Input: part model. Units: mm. Frame: model coordinates. A direction names the side the tool comes from. Give positions to 0.01 mm unless a question says otherwise; leave off trailing zeros. Loops run counter-clockwise (first coordinate to the right, second up) from the corner with the lowest first, then second, coordinate; pieces in that order, holes last. Notation, with made-up numbers: M 43.5,79 L 51.5,79 A37 cw 51.5,117 Z; hole C 39,24.25 d10. An arc over 180 degrees is marked long. Answer as a JSON object with one key per item and string values. Group by question number.
1) Section query D-D on z = 15. Return loops of the section in (x, y), plus the area to 3 significant figures.
2) First-contact query: P1, Ø5.5, axis at y = 0, z = 0, coming from the -X side (3 decimals); P2, Ø3.5, axis at x = 2, y = 3.5, coming from the -Z side; P3, Ø3, axis at x = -1, z = -16.5, coming from the -Y side; P4, Ø3.5, axis at x = 0, z = 15, coming from the -Y side. Flat tips, straight axial feed; report the tip coordinate or a pass-through.
3) Section query C-C on x = 4.25. Return loops of the section in (y, z), plus the area to 3 significant figures.
4) Section query B-B on z = 0. Return loops of the section in (x, y).
5) Section query A-A on x = 0. Return loops of the section in (y, z).
6) Ray query, L1, parallel to Z at x = 0, y = 14.7; L2, parallel to Z at x = 3.5, y = 0; L3, parallel to X at y = 14.8, z = 15. Return the intervals inside material, ascending.
7) Draft query along X for faces 5 (the flat face through (6, 7, 0)), 6 (the flat face through (1, 16, -20)), 7 (the flat face through (0, 16, -17)). Return one class per face: +X half, -X half, draft (parallel to the pull), parting line (faces both ways), or undercut.
8) Access query for faces 1 (the flat face through (3, 14, 14)), 2 (the cylindrical face through (0.18, 5.9, -3.07)), 3 (the flat face through (0, 7, -10)), 4 (the flat face through (0, 16, 13)). Directions: +Z, -Z, +X, -X, +Y, -Y. A direction counts if a zero-diameter tool reaches every point of the face in a straight line with its end or side. Return the directions, or none.
Autodesk Inventor part; units mm, degrees
ref_plane "YZ Plane" through (0, 0, 0) normal (1, 0, 0) x (0, 1, 0)
ref_plane "XZ Plane" through (0, 0, 0) normal (0, 1, 0) x (-1, 0, 0)
ref_plane "XY Plane" through (0, 0, 0) normal (0, 0, 1) x (1, 0, 0)
sketch "Sketch1" plane through (0, 0, 0) normal (1, 0, 0) x (0, 1, 0)
  line L0 (0, 0) -> (14, 0) construction
  line L1 (0, -10) -> (14, -10)
  line L2 (14, 10) -> (0, 10)
  arc A0 (0, 10) -> (0, -10) centre (0, 0) ccw
  arc A1 (14, -10) -> (14, 10) centre (14, 0) ccw construction
  line L3 (14, 10) -> (14, -10)
  point P0 (7, 0)
  dimension "d2" = 20
  dimension "d1" = 14
extrude "Extrusion1" add sketch "Sketch1" along normal mid plane 10
sketch "Sketch2" plane through (-5, 14, 10) normal (0, 1, 0) x (1, 0, 0)
  line L0 (0, -10) -> (10, -10)
  line L1 (10, -10) -> (10, 30)
  line L2 (10, 30) -> (0, 30)
  line L3 (0, 30) -> (0, -10)
  line L4 (0, 0) -> (0, 20) construction
  line L5 (0, 20) -> (10, 20) construction
  line L6 (10, 20) -> (10, 0) construction
  line L7 (10, 0) -> (0, 0) construction
  line L8 (0, 0) -> (0, 20) construction
  line L9 (10, 20) -> (10, 0) construction
  line L10 (0, 10) -> (10, 10) construction
  point P0 (5, 10)
  dimension "d28" = 40
extrude "Extrusion2" add sketch "Sketch2" along normal blind 4
sketch "Sketch3" plane through (-5, 14, 10) normal (0, -1, 0) x (1, 0, 0)
  line L0 (10, -30) -> (0, -30)
  line L1 (0, -30) -> (0, -20)
  line L2 (0, -20) -> (0, 0)
  line L3 (0, 0) -> (0, 10)
  line L4 (0, 10) -> (10, 10)
  line L5 (10, 10) -> (10, 0)
  line L6 (10, 0) -> (10, -20)
  line L7 (10, -20) -> (10, -30)
  line L8 (10, -20) -> (0, -20)
  line L9 (0, 0) -> (10, 0)
  line L10 (0, 10) -> (10, 10)
  point P0 (5, -10)
  point P1 (5, 5)
  point P2 (5, -25)
  point P3 (5, 10)
  point P4 (5, 10)
  point P5 (5, 10)
  dimension "d30" = 5
  dimension "d31" = 5
hole "Hole1" at (0, 14, 15) at (0, 14, -15) direction (0, 1, 0) diameter 3.4 end through all counterbore diameter 6 counterbore depth 2
sketch "Sketch5" plane through (5, 0, 0) normal (1, 0, 0) x (0, 0, -1)
  arc A0 (-10, 0) -> (10, 0) centre (0, 0) ccw
hole "Hole3" at (5, 0, 0) direction (-1, 0, 0) diameter 13 end through all
thicken "Thicken1" operation add thickness 0.15 both sides no extend neighbours yes toward (0, 0.0804666, -0.9967573) faces at (1.6667, 0.523, -6.4789)
sketch "Sketch6" plane through (5, 0, 0) normal (1, 0, 0) x (0, 0, -1)
  circle A0 centre (0, 0) radius 6.65 construction
  line L0 (20, 18) -> (20, 14)
  line L1 (20, 14) -> (10, 14)
  line L2 (10, 14) -> (10, 0)
  arc A1 (-10, 0) -> (10, 0) centre (0, 0) ccw
  line L3 (-10, 0) -> (-10, 14)
  line L4 (-10, 14) -> (-20, 14)
  line L5 (-20, 14) -> (-20, 18)
  line L6 (-20, 18) -> (20, 18)
  circle A2 centre (0, 0) radius 6.65
  line L7 (20, 18) -> (20, 14)
  line L8 (20, 14) -> (10, 14)
  line L9 (10, 14) -> (10, 0)
  arc A3 (-10, 0) -> (10, 0) centre (0, 0) ccw
  line L10 (-10, 0) -> (-10, 14)
  line L11 (-10, 14) -> (-20, 14)
  line L12 (-20, 14) -> (-20, 18)
  line L13 (-20, 18) -> (20, 18)
  circle A4 centre (0, 0) radius 4.65
  dimension "d37" = 2
extrude "Extrusion3" add sketch "Sketch6" along normal blind 1 contours L0 L1 L2 A1 L3 L4 L5 L6 | A2
chamfer "Chamfer2" distance 0.5 angle 45 1 edges at (-5, 0, 6.65)
chamfer "Chamfer3" distance 1 angle 45 1 edges at (6, 18, 0)
equation "\"d21\" = diameter"
equation "\"diameter\" = 13"
properties part number "bearing holder"
Output:
{
 "1": {"outline": "M -5,14 L -3,14 L -3,16 L -1.7,16 L -1.7,18 L -5,18 Z; M 1.7,16 L 3,16 L 3,14 L 6,14 L 6,17 L 5,18 L 1.7,18 Z", "area": "24.7 mm^2"},
 "2": {"P1": "passes through", "P2": "stops at z = -10", "P3": "stops at y = 14", "P4": "stops at y = 16"},
 "3": {"outline": "M 0,-10 L 14,-10 L 14,-20 L 18,-20 L 18,20 L 14,20 L 14,10 L 0,10 A10 ccw Z; hole C 0,0 d13.3", "area": "458 mm^2"},
 "4": {"outline": "M -5,-10 L 6,-10 L 6,-4.65 L 5,-4.65 L 5,-6.65 L -4.5,-6.65 L -5,-7.15 Z; M -5,7.15 L -4.5,6.65 L 5,6.65 L 5,4.65 L 6,4.65 L 6,17 L 5,18 L -5,18 Z"},
 "5": {"outline": "M 0,-10 L 14,-10 L 14,-12 L 16,-12 L 16,-13.3 L 18,-13.3 L 18,13.3 L 16,13.3 L 16,12 L 14,12 L 14,10 L 0,10 A10 ccw Z; M 14,-20 L 18,-20 L 18,-16.7 L 16,-16.7 L 16,-18 L 14,-18 Z; M 14,18 L 16,18 L 16,16.7 L 18,16.7 L 18,20 L 14,20 Z; hole C 0,0 d13.3"},
 "6": {"L1": "z = -20 to -18, -12 to 12, 18 to 20", "L2": "z = -10 to -6.65, 6.65 to 10", "L3": "x = -5 to -3, 3 to 6"},
 "7": {"face 5": "+X half", "face 6": "draft", "face 7": "undercut"},
 "8": {"face 1": "+Z, +X, -X, -Y", "face 2": "-X", "face 3": "-Z, +X, -X, -Y", "face 4": "-Y"}
}
